```python
from build123d import *

# Parameters (mm, degrees)
SKETCH2_R           = 12.658951853
BOSS_EXTRUDE4_DEPTH = 622.3


with BuildPart() as part:
    # Sketch2 → Boss-Extrude4 (new body)
    with BuildSketch(Plane.XY):
        with Locations((-46.573237559, 9.77124788)):
            Circle(SKETCH2_R)
        Polygon((-43.103074761, 15.798372741), (-50.057799401, 15.790059449), (-53.5279622, 9.762934589), (-50.043400358, 3.744123019), (-43.088675718, 3.752436311), (-39.618512919, 9.779561172), align=None, mode=Mode.SUBTRACT)
    extrude(amount=BOSS_EXTRUDE4_DEPTH)


solid = part.part
```
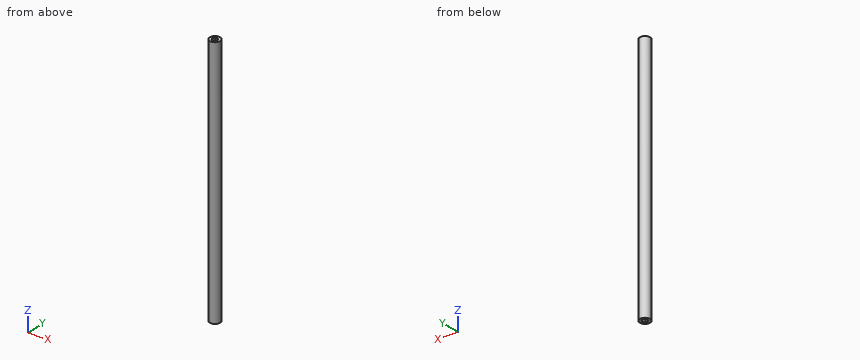
Geometry: final body of the model. Coordinates: model frame, mm. Round coordinates to 2 decimals unless told otherwise and drop trailing zeros. Write each loop counter-clockwise with the first axis right and the second up, starting at its lowest first coordinate (ties: lowest second). Pieces come first, ordered by that corner, then holes. Notation, with made-up numbers: (-4, 67.25) -> (2, 67.25) arc R14 ccw to (2, 79.25) -> close; hole circle Ø11 at (80.25, -5.75). An arc over 180 degrees is marked (long way). Return JSON: item names as keys, results as strings.
Q1. First-contact query: pin 1 Ø4 at (x, z) = (-38.5, 308) entering from +Y; pin 2 Ø3 at (x, z) = (-37, 298) entering from -Y; pin 3 Ø2 at (x, y) = (-51, 6.5) entering from -Z; pin 4 Ø5 at (y, z) = (15.5, 369.5) entering from +X. Flat tips, straight axial feed; report the tip coordinate or a pass-through.
From the geometry:
{"pin 1": "y = 20.88", "pin 2": "y = 0.02", "pin 3": "z = 0", "pin 4": "x = -34.33"}
Q2. Section A-A on z = 167.5. Return the cut outline in (x, y), and give its area (3 significant figures).
From the geometry:
{"outline": "circle Ø25.32 at (-46.57, 9.77); hole (-53.53, 9.76) -> (-50.04, 3.74) -> (-43.09, 3.75) -> (-39.62, 9.78) -> (-43.1, 15.8) -> (-50.06, 15.79) -> close", "area": "378 mm2"}
Q3. Ray query, line 1 (Y direction, x = -47.75, z = 186); line 2 (X direction, y = 15.25, z = 205); line 3 (Y direction, x = -52.75, z = 537.5). Return the intervals inside material, ascending.
From the geometry:
{"line 1": "-2.83 to 3.75, 15.79 to 22.38", "line 2": "-57.99 to -50.37, -42.79 to -35.16", "line 3": "-1.28 to 8.42, 11.11 to 20.82"}
